Design review of the part built by this model. Coordinates are the model's own, in mm. Round coordinates to 2 decimals unless told otherwise and drop trailing zeros. Loops run counter-clockwise (first coordinate to the right, second up) from the corner with the lowest first, then second, coordinate; pieces in that order, holes last. Notation, with made-up numbers: (-20.75, -15) - (-7.75, -15) arc R30 cw to (-7.75, 9) - close; hole circle Ø10 at (11.5, 89). An arc over 180 degrees is marked (long way). One line per question, with ' | ' between items. Start each with the question number.
from build123d import *

# Parameters (mm, degrees)
SKETCH1_R           = 2.5
BOSS_EXTRUDE1_DEPTH = 1.75


with BuildPart() as part:
    # Sketch1 → Boss-Extrude1 (new, symmetric)
    with BuildSketch(Plane(origin=(0, 0, 0), x_dir=(1, 0, 0), z_dir=(0, 1, 0))):
        Polygon((0, 5.196152423), (-4.5, 2.598076211), (-4.5, -2.598076211), (0, -5.196152423), (4.5, -2.598076211), (4.5, 2.598076211), align=None)
        with Locations(Location((0, 0, 0), (0, 0, 270))):
            Circle(SKETCH1_R, mode=Mode.SUBTRACT)
    extrude(amount=BOSS_EXTRUDE1_DEPTH, both=True)

    # Cut-Sweep1: sweep along a path in Sketch2
    with BuildLine(Plane(origin=(0, 1.75, 0), x_dir=(1, 0, 0), z_dir=(0, 1, 0))) as cut_sweep1_path:
        CenterArc((0, 0), 4.5, 0, 360)
    # Sketch3 → Cut-Sweep1 (sweep, cut)
    with BuildSketch(Plane.XY):
        Polygon((-5.25, 1), (-4.5, 1.75), (-5.25, 1.75), align=None)
    cut_sweep1 = sweep(path=cut_sweep1_path.line, mode=Mode.SUBTRACT)

    # Mirror1: Cut-Sweep1 across plane
    add(cut_sweep1.mirror(Plane.ZX), mode=Mode.SUBTRACT)


solid = part.part
1. Clearance check with flat-ended pins moving along their axes: P1, Ø2, axis at x = -2.5, y = 1, coming from the -Z side; P2, Ø3, axis at x = -0.5, z = -1.5, coming from the +Y side; P3, Ø2, axis at y = 1, z = 4, coming from the +X side. State where each tip first meets the part, or that it passes through.
2. Take a section at A-A, the plane y = 0.7. Give the boundary of the cut face in (x, z).
3. Take a section at B-B, the plane y = 1.3. Give the boundary of the cut face in (x, z), then the cut area to 3 significant figures.
4. The part is to be moulded in two halves that separate along X. For faces 1 (the face through (-2.44, -0.02, -0.54)), 2 (the face through (-4.04, 1.58, -2.34)), 3 (the face through (2, 1.75, 2)), say which applies: pulls with the +X half, pulls with the -X half, needs draft (parallel to the pull), parting line crosses it, or undercut.
5. To check wall thickness, follow line 1 along X through (y, z) = (1.1, 0.5); line 2 along Z through (x, y) = (1.75, 1.4); line 3 along Z through (x, y) = (-1.25, -0.65). State the ranges of each line that lie inside material, in increasing order.
Answer list:
1) P1: stops at z = -4.33 | P2: stops at y = 1.75 | P3: stops at x = 3.8
2) outline: (-4.5, -2.6) - (0, -5.2) - (4.5, -2.6) - (4.5, 2.6) - (0, 5.2) - (-4.5, 2.6) - close; hole circle Ø5 at (0, 0)
3) outline: (-4.5, -2.06) arc R4.95 ccw to (-4.04, -2.87) - (-0.46, -4.93) arc R4.95 ccw to (0.46, -4.93) - (4.04, -2.87) arc R4.95 ccw to (4.5, -2.06) - (4.5, 2.06) arc R4.95 ccw to (4.04, 2.87) - (0.46, 4.93) arc R4.95 ccw to (-0.46, 4.93) - (-4.04, 2.87) arc R4.95 ccw to (-4.5, 2.06) - close; hole circle Ø5 at (0, 0) | area: 49.8 mm²
4) face 1: undercut | face 2: pulls with the -X half | face 3: needs draft
5) line 1: x = -4.5 to -2.45, 2.45 to 4.5 | line 2: z = -4.19 to -1.79, 1.79 to 4.19 | line 3: z = -4.47 to -2.17, 2.17 to 4.47
